from build123d import *

# Parameters (mm, degrees)
BOSS_EXTRUDE1_DEPTH = 15
SKETCH3_R           = 2.5
BOSS_EXTRUDE2_DEPTH = 2
SKETCH5_R           = 0.5
CUT_EXTRUDE1_DEPTH  = 24.086792761
FILLET1_R           = 0.1


with BuildPart() as part:
    # Sketch1 → Boss-Extrude1 (new body)
    with BuildSketch(Plane.XY):
        with BuildLine():
            Line((0, 2.5), (0, 9.5))
            ThreePointArc((0, 9.5), (5, 12), (10, 9.5))
            Line((10, 9.5), (10, 2.5))
            ThreePointArc((10, 2.5), (5, 0), (0, 2.5))
        make_face()
    extrude(amount=-BOSS_EXTRUDE1_DEPTH)

    # Sketch3 → Boss-Extrude2 (add)
    with BuildSketch(Plane(origin=(0, 0, -15), x_dir=(-1, 0, 0), z_dir=(0, 0, -1))):
        with Locations(Location((-5, 6, 0), (0, 0, 180))):
            Circle(SKETCH3_R)
    extrude(amount=BOSS_EXTRUDE2_DEPTH)

    # Sketch5 → Cut-Extrude1 (cut, through all)
    with BuildSketch(Plane(origin=(0, 0, -17), x_dir=(-1, 0, 0), z_dir=(0, 0, -1))):
        with Locations((-5, 6)):
            Circle(SKETCH5_R)
    extrude(amount=-CUT_EXTRUDE1_DEPTH, mode=Mode.SUBTRACT)

    # Fillet1
    fillet1_edges = [part.edges().sort_by_distance(p)[0] for p in [
        (2.5, 6, -15),
        (2.5, 6, -17),
    ]]
    fillet(fillet1_edges, radius=FILLET1_R)


solid = part.part
Check sheet for the modelled part. Datum: model origin and axes. Units: mm. A direction names the side the tool comes from. Coordinates: 2 decimals unless noted, no trailing zeros. Loops run counter-clockwise (first coordinate to the right, second up) from the corner with the lowest first, then second, coordinate; pieces in that order, holes last. Notation, with made-up numbers: (65.5, 31) -> (89.5, 31) arc R12 ccw to (89.5, 48) -> close; hole circle Ø9 at (39.25, 18). An arc over 180 degrees is marked (long way). Write item = value, one per line. Start each with the question number.
1. Material ranges on line 1 (Y direction, x = 5, z = -11.5); line 2 (Z direction, x = 4.5, y = 10.75); line 3 (Y direction, x = 3.25, z = -8), recorded low to high.
2. Section check C-C on z = -11.5. Record the cut outline in (x, y), then the cut area to 3 significant figures.
3. Draft check along X on faces 1 (the flat face through (0, 6, -7)), 2 (the flat face through (5, 9, -15)), 3 (the cylindrical face through (5.4, 5.7, -8.6)), 4 (the flat face through (10, 6, -7)). Enter one of: released by +X, released by -X, zero draft, split by the parting line, or undercut.
4. Section check D-D on y = 1.25. Record the cut outline in (x, z), then the cut area to 4 significant figures.
5. Depth check by flat-ended pin: P1, Ø1, axis at x = 6.5, y = 2.5, coming from the -Z side. Enter the tip coordinate at first touch or a pass-through.
6. Section check A-A on y = 6. Record the cut outline in (x, z), then the cut area to 3 significant figures.
7. Section check B-B on x = 5. Record the cut outline in (y, z).
8. Tool access check on faces 5 (the cylindrical face through (5, 0, -7)), 6 (the cylindrical face through (7.385, 5.249, -15.987)). Record the directions out of +Z, -Z, +X, -X, +Y, -Y that give a thin tool (end or side, any length) a straight path to the whole face; none if there is none.
Responses:
q1.line_1 = 0 to 5.5, 6.5 to 12
q1.line_2 = -15 to 0
q1.line_3 = 0.25 to 11.75
q2.outline = (0, 2.5) arc R6.25 ccw to (10, 2.5) -> (10, 9.5) arc R6.25 ccw to (0, 9.5) -> close; hole circle Ø1 at (5, 6)
q2.area = 104 mm2
q3.face_1 = released by -X
q3.face_2 = zero draft
q3.face_3 = undercut
q3.face_4 = released by +X
q4.outline = (1.25, -15) -> (8.75, -15) -> (8.75, 0) -> (1.25, 0) -> close
q4.area = 112.5 mm2
q5.P1 = -15
q6.outline = (0, -15) -> (2.4, -15) arc R0.1 cw to (2.5, -15.1) -> (2.5, -16.9) arc R0.1 ccw to (2.6, -17) -> (4.5, -17) -> (4.5, 0) -> (0, 0) -> close; (5.5, -17) -> (7.4, -17) arc R0.1 ccw to (7.5, -16.9) -> (7.5, -15.1) arc R0.1 cw to (7.6, -15) -> (10, -15) -> (10, 0) -> (5.5, 0) -> close
q6.area = 143 mm2
q7.outline = (0, -15) -> (3.4, -15) arc R0.1 cw to (3.5, -15.1) -> (3.5, -16.9) arc R0.1 ccw to (3.6, -17) -> (5.5, -17) -> (5.5, 0) -> (0, 0) -> close; (6.5, -17) -> (8.4, -17) arc R0.1 ccw to (8.5, -16.9) -> (8.5, -15.1) arc R0.1 cw to (8.6, -15) -> (12, -15) -> (12, 0) -> (6.5, 0) -> close
q8.face_5 = +Z, -Z, -Y
q8.face_6 = -Z
